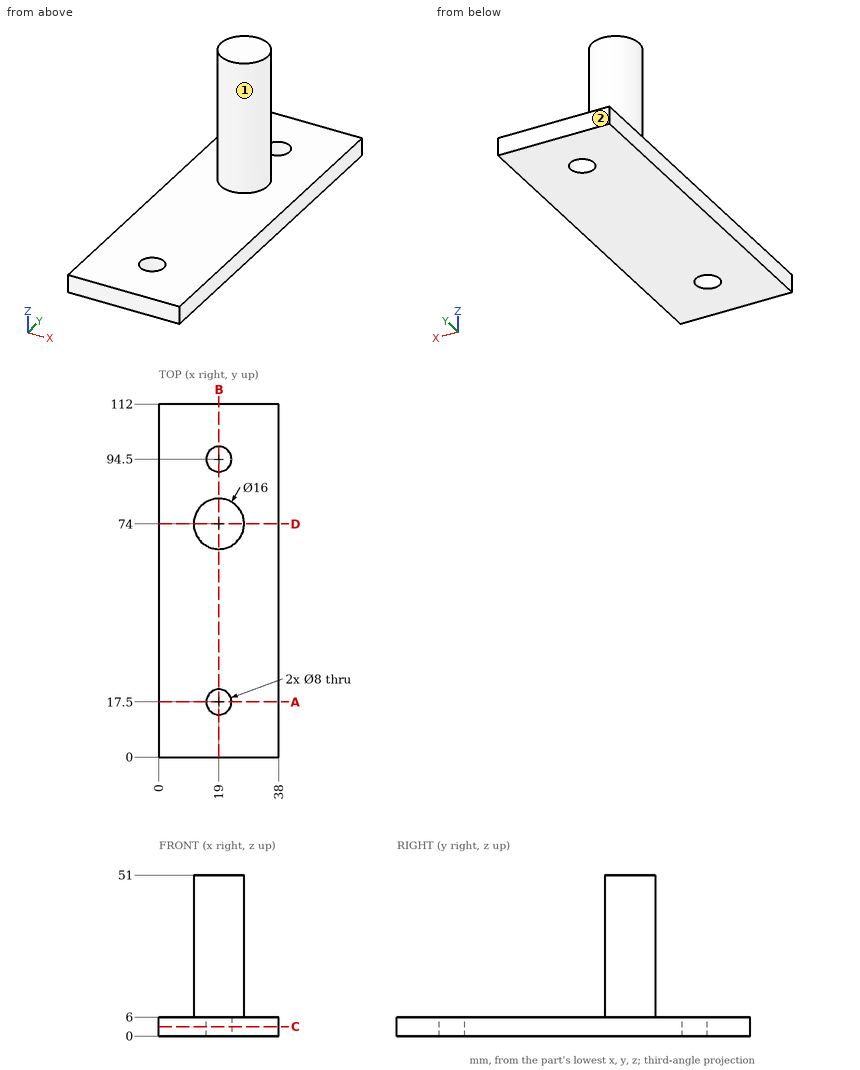
Design review of the part shown in the three views and the two pictorial views. Dimensions are in mm from the part's minimum x, y and z. A direction names the side the tool comes from. Give positions to 0.01 mm unless a question says otherwise; leave off trailing zeros. Order: outer loops, then holes, each group sorted by start corner. A loop starts at its lowest first (then second) coordinate and runs counter-clockwise, first axis right, second up. Notation, with made-up numbers: M 33.5,79 L 50.5,79 A33 ccw 50.5,114 Z; hole C 50.25,37 d2. An arc over 180 degrees is marked long. Answer in a Markdown table with one row per item. Add a question column.
(1) For pin 1 (6.5 mm diameter, centred on x = 19, y = 94.5, fed in from +Z); pin 2 (6 mm diameter, centred on x = 24.5, z = 27, fed in from +Y); pin 3 (5 mm diameter, centred on x = 5, y = 34.5, fed in from +Z); pin 4 (5 mm diameter, centred on x = 26, z = 26, fed in from -Y), all flat-tipped, find the tip position at first contact; note any pin that passes through.
(2) Consider section C-C on z = 3. State the section outline as (x, y) points.
(3) Consider section A-A on y = 17.5. State the section outline as (x, z) points.
(4) For the marked faces 1 and 2, list the 3-axis set-ups (+Z, -Z, +X, -X, +Y, -Y) from which the entire face can be reached by the end or side of a thin tool; tool diameter is ignored.
(5) Consider section B-B on x = 19. State the section outline as (y, z) points, and give its area (3 significant figures).
(6) Wall thickness on probe 1 along Y at (x, z) = (19, 4); probe 2 along Z at (x, y) = (35.5, 80); probe 3 along Y at (x, z) = (19.5, 22.5): over which ranges is each line inside the solid? List them lowest first. Write a range as [from, to].
(7) Consider section D-D on y = 74. State the section outline as (x, z) points, and give its area (3 significant figures).
Evaluation:
| question | item | result |
|---|---|---|
| 1 | pin 1 | passes through |
| 1 | pin 2 | stops at y = 81.6 |
| 1 | pin 3 | stops at z = 6 |
| 1 | pin 4 | stops at y = 67.39 |
| 2 | outline | M 0,0 L 38,0 L 38,112 L 0,112 Z; hole C 19,17.5 d8; hole C 19,94.5 d8 |
| 3 | outline | M 0,0 L 15,0 L 15,6 L 0,6 Z; M 23,0 L 38,0 L 38,6 L 23,6 Z |
| 4 | face 1 | +Z |
| 4 | face 2 | +Z, -Z, +X, -X, +Y |
| 5 | outline | M 0,0 L 13.5,0 L 13.5,6 L 0,6 Z; M 21.5,0 L 90.5,0 L 90.5,6 L 82,6 L 82,51 L 66,51 L 66,6 L 21.5,6 Z; M 98.5,0 L 112,0 L 112,6 L 98.5,6 Z |
| 5 | area | 1,300 mm^2 |
| 6 | probe 1 | y = [0, 13.5], [21.5, 90.5], [98.5, 112] |
| 6 | probe 2 | z = [0, 6] |
| 6 | probe 3 | y = [66.02, 81.98] |
| 7 | outline | M 0,0 L 38,0 L 38,6 L 27,6 L 27,51 L 11,51 L 11,6 L 0,6 Z |
| 7 | area | 948 mm^2 |
